from build123d import *

# Parameters (mm, degrees)
ESQUISSE1_R                  = 19.25
ESQUISSE1_R_2                = 2.5
BOSS_EXTRU_1_DEPTH           = 42
ENL_V_MAT_EXTRU_1_DEPTH      = 74.881298321
ENL_V_MAT_EXTRU_1_DEPTH_BACK = 74.881298321
ESQUISSE2_W                  = 90
ESQUISSE2_H                  = 30
ESQUISSE3_R                  = 1
ENL_V_MAT_EXTRU_2_DEPTH      = 42
ENL_V_MAT_EXTRU_3_DEPTH      = 78.729096869
ENL_V_MAT_EXTRU_3_DEPTH_BACK = 78.729096869
ESQUISSE4_W                  = 87.75
ESQUISSE4_H                  = 39


with BuildPart() as part:
    # Esquisse1 → Boss.-Extru.1 (new body)
    with BuildSketch(Plane.XY):
        with BuildLine():
            Line((12.13875, 26.612276273), (53.5275, 7.733481994))
            ThreePointArc((53.5275, 7.733481994), (58.5, 0), (53.5275, -7.733481994))
            Line((53.5275, -7.733481994), (12.13875, -26.612276273))
            ThreePointArc((12.13875, -26.612276273), (-29.25, 0), (12.13875, 26.612276273))
        make_face()
        with Locations(Location((0, 0, 0), (0, 0, 180))):
            Circle(ESQUISSE1_R, mode=Mode.SUBTRACT)
        with Locations(Location((50, 0, 0), (0, 0, 180))):
            Circle(ESQUISSE1_R_2, mode=Mode.SUBTRACT)
    extrude(amount=BOSS_EXTRU_1_DEPTH)

    # Esquisse2 → Enlèv. mat.-Extru.1 (cut, two sides: drawn at the far end of the back side and taken through both)
    with BuildSketch(Plane(origin=(5.218823759, 0, 0), x_dir=(1, 0, 0), z_dir=(0, 1, 0)).offset(-ENL_V_MAT_EXTRU_1_DEPTH_BACK)):
        with Locations((-11.691323759, -21)):
            Rectangle(ESQUISSE2_W, ESQUISSE2_H)
    extrude(amount=ENL_V_MAT_EXTRU_1_DEPTH + ENL_V_MAT_EXTRU_1_DEPTH_BACK, mode=Mode.SUBTRACT)

    # Esquisse3 → Enlèv. mat.-Extru.2 (cut)
    with BuildSketch(Plane.XY.offset(42)):
        with Locations((45, 5)):
            Circle(ESQUISSE3_R)
        with Locations((45, -5)):
            Circle(ESQUISSE3_R)
        with Locations((-15, 19)):
            Circle(ESQUISSE3_R)
        with Locations((-15, -19)):
            Circle(ESQUISSE3_R)
    extrude(amount=-ENL_V_MAT_EXTRU_2_DEPTH, mode=Mode.SUBTRACT)

    # Esquisse4 → Enlèv. mat.-Extru.3 (cut, two sides: drawn at the far end of the back side and taken through both)
    with BuildSketch(Plane(origin=(0, 0, 0), x_dir=(1, 0, 0), z_dir=(0, 1, 0)).offset(-ENL_V_MAT_EXTRU_3_DEPTH_BACK)):
        with Locations((14.625, -22.5)):
            Rectangle(ESQUISSE4_W, ESQUISSE4_H)
    extrude(amount=ENL_V_MAT_EXTRU_3_DEPTH + ENL_V_MAT_EXTRU_3_DEPTH_BACK, mode=Mode.SUBTRACT)


solid = part.part
Build history of the part. All positions in model axes, mm. Coordinates: 2 decimals unless noted, no trailing zeros. Order: outer loops, then holes, each group sorted by start corner. A loop starts at its lowest first (then second) coordinate and runs counter-clockwise, first axis right, second up. Notation, with made-up numbers: (21, 6.5) - (65, 6.5) arc R20 cw to (65, 20.5) - close; hole circle Ø3 at (0, -38). An arc over 180 degrees is marked (long way). Write each question's results on one line, items separated by ' | '. Start each with the question number.
Item 1: Wall check: probe 1 along Y at (x, z) = (0, 1.85); probe 2 along Y at (x, z) = (45, 1.15); probe 3 along X at (y, z) = (1.5, 0.85). Give the ranges that are in metal, low to high. Write a range as [from, to].
Item 2: Flat gauge pins, fed straight in: pin 1 (1.5 mm diameter, centred on y = 22.5, z = 0.5, fed in from +X); pin 2 (2.5 mm diameter, centred on x = -15, y = -19, fed in from -Z); pin 3 (3 mm diameter, centred on x = -12, y = 11.5, fed in from -Z). Where does each tip first touch, or does it go through?
Item 3: Band-saw the part on B-B on z = 2.15. Write the cut outline in (x, y).
Item 4: Mould opens along X. For faces 1 (the face through (25, 0, 0)), 2 (the face through (15.28, 11.71, 1.48)), 3 (the face through (-29.24, -0.82, 1.48)) say: released by +X, released by -X, zero draft, split by the parting line, or undercut.
Item 5: Band-saw the part on A-A on y = 0. Write the cut outline in (x, z), and give its area (3 significant figures).
Item 6: Band-saw the part on D-D on y = -10.5. Write the cut outline in (x, z), and give its area (3 significant figures).
Item 7: Band-saw the part on C-C on x = 0. Write the cut outline in (y, z), and give its area (3 significant figures).
Numbers:
1) probe 1: [-29.25, -19.25], [19.25, 29.25] | probe 2: [-11.62, -6], [-4, 4], [6, 11.62] | probe 3: [-29.21, -19.19], [19.19, 48], [52, 58.37]
2) pin 1: x = 22.8 | pin 2: z = 0 | pin 3: through
3) outline: (12.14, -26.61) - (53.53, -7.73) arc R8.5 ccw to (53.53, 7.73) - (12.14, 26.61) arc R29.25 ccw (long way) to start; hole circle Ø38.5 at (0, 0); hole circle Ø2 at (-15, -19); hole circle Ø2 at (-15, 19); hole circle Ø2 at (45, -5); hole circle Ø2 at (45, 5); hole circle Ø5 at (50, 0)
4) face 1: zero draft | face 2: undercut | face 3: split by the parting line
5) outline: (-29.25, 0) - (-19.25, 0) - (-19.25, 3) - (-29.25, 3) - close; (19.25, 0) - (47.5, 0) - (47.5, 3) - (19.25, 3) - close; (52.5, 0) - (58.5, 0) - (58.5, 3) - (52.5, 3) - close | area: 133 mm^2
6) outline: (-27.3, 0) - (-16.13, 0) - (-16.13, 3) - (-27.3, 3) - close; (16.13, 0) - (47.46, 0) - (47.46, 3) - (16.13, 3) - close | area: 127 mm^2
7) outline: (-29.25, 0) - (-19.25, 0) - (-19.25, 3) - (-29.25, 3) - close; (19.25, 0) - (29.25, 0) - (29.25, 3) - (19.25, 3) - close | area: 60.0 mm^2
